The model under review builds one solid part; all positions refer to its coordinate system, in mm. A direction names the side the tool comes from. Coordinates: 2 decimals unless noted, no trailing zeros. Write each loop counter-clockwise with the first axis right and the second up, starting at its lowest first coordinate (ties: lowest second). Pieces come first, ordered by that corner, then holes.
```python
from build123d import *

# Parameters (mm, degrees)
BOSS_EXTRUDE2_DEPTH     = 8.3
CIRPATTERN1_COUNT       = 4
SKETCH13_R              = 22.4
CUT_EXTRUDE3_DEPTH      = 4
FILLET1_R               = 5
SKETCH15_R              = 18
SKETCH15_R_2            = 15
BOSS_EXTRUDE3_DEPTH     = 4
SKETCH16_R              = 7.5
CUT_EXTRUDE4_DEPTH      = 103.587698187
FILLET2_R               = 5
FILLET4_R               = 3
FILLET5_R               = 2
FILLET6_R               = 2
TAP_DRILL_FOR_M6_TAP1_D = 5


with BuildPart() as part:
    # Sketch1 → Revolve1 (revolve)
    with BuildSketch(Plane.XY, mode=Mode.PRIVATE) as revolve1_sk:
        Polygon((22.3, -26.9), (53.8, -26.9), (53.8, 0.95810827), (56.6, 0.95810827), (56.6, 3.75810827), (59, 3.75810827), (59, 0), (59, -31.9), (0, -31.9), (0, -26.9), (17.5, -26.9), (17.5, -6.8), (22.3, -6.8), align=None)
    revolve(revolve1_sk.sketch.rotate(Axis((0, -26.9, 0), (0, -1, 0)), 180), axis=Axis((0, -26.9, 0), (0, -1, 0)))

    # Sketch2 → Boss-Extrude2 (add)
    with BuildSketch(Plane(origin=(0, 3.75810827, 0), x_dir=(1, 0, 0), z_dir=(0, 1, 0))):
        Polygon((7.756499668, 69), (-8.243500332, 69), (-11.893500332, 57.788793462), (11.406499668, 57.88688768), align=None)
    boss_extrude2 = extrude(amount=-BOSS_EXTRUDE2_DEPTH)

    # CirPattern1: Boss-Extrude2 ×4 about axis
    cirpattern1_axis = Axis((0, 0, 0), (0, 1, 0))
    for i in range(1, CIRPATTERN1_COUNT):
        add(boss_extrude2.rotate(cirpattern1_axis, i * 360 / CIRPATTERN1_COUNT))

    # Sketch10 → Cut-Revolve4 (revolve, cut)
    with BuildSketch(Plane(origin=(0, 0, 0), x_dir=(0, 0, -1), z_dir=(1, 0, 0)), mode=Mode.PRIVATE) as cut_revolve4_sk:
        Polygon((59.74122217, -25.056663082), (55.637901582, -24.521737202), (54.676040662, -31.9), (59.74122217, -32.409345916), align=None)
    revolve(cut_revolve4_sk.sketch.rotate(Axis((0, -1.306352148, 0), (0, -1, 0)), 281.147212692), axis=Axis((0, -1.306352148, 0), (0, -1, 0)), mode=Mode.SUBTRACT)

    # Sketch8 → Cut-Revolve5 (revolve, cut)
    with BuildSketch(Plane(origin=(0, 0, 0), x_dir=(0, 0, -1), z_dir=(1, 0, 0)), mode=Mode.PRIVATE) as cut_revolve5_sk:
        Polygon((57.88688768, -4.54189173), (59, -4.54189173), (59, -31.9), (56, -31.9), align=None)
    revolve(cut_revolve5_sk.sketch.rotate(Axis((0, 5.358719866, 0), (0, -1, 0)), 180), axis=Axis((0, 5.358719866, 0), (0, -1, 0)), mode=Mode.SUBTRACT)

    # Sketch12 → Cut-Revolve6 (revolve, cut)
    with BuildSketch(Plane(origin=(0, 0, 0), x_dir=(0, 0, -1), z_dir=(1, 0, 0))):
        Polygon((-55.049732908, -31.9), (-54.904154696, -30.15017811), (-17.788536772, -31.9), align=None)
    revolve(axis=Axis((0, 13.859698408, 0), (0, -1, 0)), mode=Mode.SUBTRACT)

    # Sketch13 → Cut-Extrude3 (cut)
    with BuildSketch(Plane.XZ.offset(31.9)):
        Circle(SKETCH13_R)
    extrude(amount=-CUT_EXTRUDE3_DEPTH, mode=Mode.SUBTRACT)

    # Fillet1
    # the kernel refuses this fillet: 5 mm, written as the material it takes off along each edge
    with BuildSketch(Plane(origin=(0, -31.68259181, 0), x_dir=(0, 0, 1), z_dir=(1, 0, 0))) as fillet1_piece_1:
        with BuildLine():
            CenterArc((27.185563904, -5.231169776), FILLET1_R, 87.300779723, 75.858290504)
            Line((22.4, -3.78259181), (22.304288722, -3.753620251))
            ThreePointArc((22.304288722, -3.753620251), (22.3, -1.891295905), (22.3, 0))
            Line((22.3, 0), (22.404709286, 0.099889052))
            Line((22.404709286, 0.099889052), (27.425737475, -0.136828145))
            Line((27.425737475, -0.136828145), (27.421028189, -0.236717197))
        make_face()
    revolve(axis=Axis((0, -31.68259181, 0), (0, -1, 0)), revolution_arc=270, mode=Mode.SUBTRACT)
    with BuildSketch(Plane(origin=(0, -31.68259181, 0), x_dir=(1, 0, 0), z_dir=(0, 0, -1))) as fillet1_piece_2:
        with BuildLine():
            CenterArc((27.185563904, -5.231169776), FILLET1_R, 87.300779723, 75.858290504)
            Line((22.4, -3.78259181), (22.304288722, -3.753620251))
            ThreePointArc((22.304288722, -3.753620251), (22.3, -1.891295905), (22.3, 0))
            Line((22.3, 0), (22.404709286, 0.099889052))
            Line((22.404709286, 0.099889052), (27.425737475, -0.136828145))
            Line((27.425737475, -0.136828145), (27.421028189, -0.236717197))
        make_face()
    revolve(axis=Axis((0, -31.68259181, 0), (0, -1, 0)), revolution_arc=90, mode=Mode.SUBTRACT)

    # Sketch15 → Boss-Extrude3 (add)
    with BuildSketch(Plane.XZ.offset(27.9)):
        Circle(SKETCH15_R)
        Circle(SKETCH15_R_2, mode=Mode.SUBTRACT)
    extrude(amount=BOSS_EXTRUDE3_DEPTH)

    # Sketch16 → Cut-Extrude4 (cut, through all)
    with BuildSketch(Plane.XZ.offset(27.9)):
        Circle(SKETCH16_R)
    extrude(amount=-CUT_EXTRUDE4_DEPTH, mode=Mode.SUBTRACT)

    # Fillet2
    fillet2_edges = [part.edges().sort_by_distance(p)[0] for p in [
        (-22.4, -27.9, 0),
    ]]
    fillet(fillet2_edges, radius=FILLET2_R)

    # Fillet4
    fillet4_edges = [part.edges().sort_by_distance(p)[0] for p in [
        (11.406499668, -0.39189173, -57.88688768),
        (-11.893500332, -0.39189173, -57.788793462),
        (-57.88688768, -0.39189173, -11.406499668),
        (-57.788793462, -0.39189173, 11.893500332),
        (-11.406499668, -0.39189173, 57.88688768),
        (11.893500332, -0.39189173, 57.788793462),
        (57.88688768, -0.39189173, 11.406499668),
        (57.788793462, -0.39189173, -11.893500332),
    ]]
    fillet(fillet4_edges, radius=FILLET4_R)

    # Fillet5
    fillet5_edges = [part.edges().sort_by_distance(p)[0] for p in [
        (-8.243500332, -0.39189173, -69),
        (7.756499668, -0.39189173, -69),
        (-69, -0.39189173, 8.243500332),
        (-69, -0.39189173, -7.756499668),
        (8.243500332, -0.39189173, 69),
        (-7.756499668, -0.39189173, 69),
        (69, -0.39189173, -8.243500332),
        (69, -0.39189173, 7.756499668),
    ]]
    fillet(fillet5_edges, radius=FILLET5_R)

    # Fillet6
    # the kernel refuses this fillet: 2 mm, written as the material it takes off along each edge
    with BuildSketch(Plane(origin=(0, -24.634269562, 0), x_dir=(0, 0, 1), z_dir=(-1, 0, 0))) as fillet6_piece_1:
        with BuildLine():
            CenterArc((54.622986935, 1.835886142), FILLET6_R, 300.494611252, 55.559949074)
            Line((55.637901582, 0.112532359), (55.658199875, 0.078065284))
            ThreePointArc((55.658199875, 0.078065284), (56.064338554, 0.016601804), (56.495946338, -0.039664376))
            Line((56.495946338, -0.039664376), (56.541022351, -0.00275226))
            Line((56.541022351, -0.00275226), (56.658152184, 1.695520873))
            Line((56.658152184, 1.695520873), (56.618246983, 1.698273133))
        make_face()
    revolve(axis=Axis((0, -24.634269562, 0), (0, 1, 0)), revolution_arc=258.852787308, mode=Mode.SUBTRACT)
    with BuildSketch(Plane(origin=(0, -24.634269562, 0), x_dir=(-0.9811336895007642, 0, -0.1933305028354758), z_dir=(0.1933305028354758, 0, -0.9811336895007642))) as fillet6_piece_2:
        with BuildLine():
            CenterArc((54.622986935, 1.835886142), FILLET6_R, 300.494611252, 55.559949074)
            Line((55.637901582, 0.112532359), (55.658199875, 0.078065284))
            ThreePointArc((55.658199875, 0.078065284), (56.064338554, 0.016601804), (56.495946338, -0.039664376))
            Line((56.495946338, -0.039664376), (56.541022351, -0.00275226))
            Line((56.541022351, -0.00275226), (56.658152184, 1.695520873))
            Line((56.658152184, 1.695520873), (56.618246983, 1.698273133))
        make_face()
    revolve(axis=Axis((0, -24.634269562, 0), (0, 1, 0)), revolution_arc=101.147212692, mode=Mode.SUBTRACT)

    # Tap Drill for M6 Tap1 (through all)
    with Locations(Plane(origin=(0, 3.75810827, 0), x_dir=(1, 0, 0), z_dir=(0, 1, 0))):
        with Locations((-0.243500332, 62.31716076), (62.31716076, 0.243500332), (0.243500332, -62.31716076), (-62.31716076, -0.243500332)):
            Hole(TAP_DRILL_FOR_M6_TAP1_D / 2)


solid = part.part
```
Item 1: To check wall thickness, follow line 1 along X through (y, z) = (0, -1); line 2 along Z through (x, y) = (-13, -23.5); line 3 along X through (y, z) = (-29, -16). State the ranges of each line that lie inside material, in increasing order.
Solved:
line 1: x = -69 to -64.49, -60.15 to -53.79, 53.79 to 59.93, 64.7 to 69
line 2: z = -54.98 to -52.21, -18.12 to -11.72, 11.72 to 18.12, 52.21 to 54.98
line 3: x = -52.68 to -16.06, -8.25 to 8.25, 16.06 to 52.68
Item 2: Take a section at A-A, the plane y = -10. Write out the cut boundary in (x, z), plus the area to 3 significant figures.
Solved:
outline: circle Ø115.02 at (0, 0); circle Ø44.6 at (0, 0); hole circle Ø107.6 at (0, 0); hole circle Ø35 at (0, 0)
area: 1,900 mm2
Item 3: For pin 1 (13.5 mm diameter, centred on x = -6.5, z = 4, fed in from +Y); pin 2 (1 mm diameter, centred on y = -1, z = -16.5, fed in from +X); pin 3 (1.5 mm diameter, centred on x = -42.5, z = 21, fed in from -Y), all flat-tipped, find the tip position at first contact; note any pin that passes through.
Solved:
pin 1: stops at y = -26.9
pin 2: stops at x = 56.79
pin 3: stops at y = -30.54
Item 4: Machinability: for faces 1 (the face through (-4, -27.9, 7)), 2 (the face through (23, -26.9, -1)), 3 (the face through (10, -0.3, 63.6)), which of the approach directions +Z, -Z, +X, -X, +Y, -Y give a long, thin tool a straight path to every point of the face, cutting with its end or side? Answer none if there is none.
Solved:
face 1: -Y
face 2: +Y
face 3: +Z, +X, +Y, -Y
Item 5: Mouldability with a two-part tool opening along Z and no side actions: class faces 4 (the face through (63.6, -0.3, -10)), 5 (the face through (41.2, -4.542, -41.2)), 6 (the face through (-17.5, -27.9, -4.9)) as pulls with the +Z half, pulls with the -Z half, needs draft (parallel to the pull), parting line crosses it, or undercut.
Solved:
face 4: pulls with the -Z half
face 5: needs draft
face 6: undercut
Item 6: Take a section at B-B, the plane x = 0. Count the separate pieces of the cut face and the enclosed holes in it, plus the area to 3 significant figures.
Solved:
separate pieces: 4
enclosed holes: 0
area: 798 mm2
